Geometry check sheet. Reference: the model listing, model coordinates, mm. A direction names the side the tool comes from. Coordinates: 2 decimals unless noted, no trailing zeros. Write each loop counter-clockwise with the first axis right and the second up, starting at its lowest first coordinate (ties: lowest second). Pieces come first, ordered by that corner, then holes. Notation, with made-up numbers: (-8.75, 88) -> (46.25, 88) arc R8 cw to (46.25, 95) -> close; hole circle Ø2 at (1.5, 52.25). An arc over 180 degrees is marked (long way). Answer as CSV lines item,"result".
```python
from build123d import *

# Parameters (mm, degrees)
SKETCH1_R          = 20
EXTRUDE1_DEPTH     = 15
SKETCH2_R          = 10
EXTRUDE2_DEPTH     = 5
SKETCH3_R          = 3
CUT_EXTRUDE1_DEPTH = 35.641016151


with BuildPart() as part:
    # Sketch1 → Extrude1 (new body)
    with BuildSketch(Plane(origin=(0, 0, 0), x_dir=(1, 0, 0), z_dir=(0, 1, 0))):
        with Locations(Location((0, 0, 0), (0, 0, 270))):
            Circle(SKETCH1_R)
    extrude(amount=-EXTRUDE1_DEPTH)

    # Sketch2 → Extrude2 (add)
    with BuildSketch(Plane(origin=(0, 0, 0), x_dir=(1, 0, 0), z_dir=(0, 1, 0))):
        with Locations(Location((0, 0, 0), (0, 0, 270))):
            Circle(SKETCH2_R)
    extrude(amount=EXTRUDE2_DEPTH)

    # Sketch3 → Cut-Extrude1 (cut, through all)
    with BuildSketch(Plane(origin=(0, 5, 0), x_dir=(1, 0, 0), z_dir=(0, 1, 0))):
        with Locations(Location((0, 0, 0), (0, 0, 270))):
            Circle(SKETCH3_R)
    extrude(amount=-CUT_EXTRUDE1_DEPTH, mode=Mode.SUBTRACT)


solid = part.part
```
Item 1: Cross-section at D-D, the plane z = 7.5. Record the cut outline in (x, y).
Responses:
outline,"(-18.54, -15) -> (18.54, -15) -> (18.54, 0) -> (6.61, 0) -> (6.61, 5) -> (-6.61, 5) -> (-6.61, 0) -> (-18.54, 0) -> close"
Item 2: Cross-section at C-C, the plane y = 3.5. Record the cut outline in (x, z).
Responses:
outline,"circle Ø20 at (0, 0); hole circle Ø6 at (0, 0)"
Item 3: Cross-section at A-A, the plane x = 0. Record the cut outline in (y, z), plus the area to 3 significant figures.
Responses:
outline,"(-15, -20) -> (0, -20) -> (0, -10) -> (5, -10) -> (5, -3) -> (-15, -3) -> close; (-15, 3) -> (5, 3) -> (5, 10) -> (0, 10) -> (0, 20) -> (-15, 20) -> close"
area,"580 mm2"
Item 4: Thickness scan on probe 1 along X at (y, z) = (-3.5, 0); probe 2 along Y at (x, z) = (1, -13); probe 3 along X at (y, z) = (0.75, 0). Record the ranges inside material, lowest first.
Responses:
probe 1,"x = -20 to -3, 3 to 20"
probe 2,"y = -15 to 0"
probe 3,"x = -10 to -3, 3 to 10"
Item 5: Depth check by flat-ended pin: pin 1 Ø1 at (x, y) = (-8, -11) entering from +Z; pin 2 Ø10 at (y, z) = (-1, 4.5) entering from -X; pin 3 Ø1.5 at (x, y) = (13.5, -11.5) entering from +Z. Enter the tip coordinate at first touch or a pass-through.
Responses:
pin 1,"stops at z = 18.54"
pin 2,"stops at x = -20"
pin 3,"stops at z = 15.41"
Item 6: Set-up check for faces 4 (the flat face through (0, -15, 4)), 5 (the flat face through (9, 0, -5)): record each of +Z, -Z, +X, -X, +Y, -Y from which the full face is reachable in a straight line by a thin tool's end or side.
Responses:
face 4,"+Z, -Z, +X, -X, -Y"
face 5,"+Y"
Item 7: Cross-section at B-B, the plane z = 0. Record the cut outline in (x, y).
Responses:
outline,"(-20, -15) -> (-3, -15) -> (-3, 5) -> (-10, 5) -> (-10, 0) -> (-20, 0) -> close; (3, -15) -> (20, -15) -> (20, 0) -> (10, 0) -> (10, 5) -> (3, 5) -> close"
Item 8: Release check for a two-part mould opening along X. For faces 1 (the cylindrical face through (-9.76, 2.46, -2.17)), 2 (the flat face through (2.4, 5, 2.1)), 3 (the cylindrical face through (0.9, -4.86, 2.86)) record: +X half, -X half, draft (parallel to the pull), parting line (faces both ways), or undercut.
Responses:
face 1,"parting line"
face 2,"draft"
face 3,"undercut"
